Autodesk Inventor part; units mm, degrees
ref_plane "YZ Plane" through (0, 0, 0) normal (1, 0, 0) x (0, 1, 0)
ref_plane "XZ Plane" through (0, 0, 0) normal (0, 1, 0) x (-1, 0, 0)
ref_plane "XY Plane" through (0, 0, 0) normal (0, 0, 1) x (1, 0, 0)
ref_plane "Arbeitsebene1" through (8.2312, -3.2392, 2) normal (0, 0, 1) x (1, 0, 0)
sketch "Skizze1" plane through (8.2312, -3.2392, 2) normal (0, 0, 1) x (1, 0, 0)
  arc A0 (-29.666, 52.3362) -> (-30.2278, 49.15) centre (-26.4114, 50.1197) ccw
  line L0 (-30.4697, 49.0886) -> (-31.8651, 51.0813)
  line L1 (-27.3731, 44.6661) -> (-28.7684, 46.6589)
  line L2 (-25.3803, 46.0614) -> (-27.3731, 44.6661)
  spline S0 degree 3 poles (-25.3803, 46.0614) (-25.4758, 46.0372) (-25.5717, 46.0164) (-25.765, 45.9815) (-25.8623, 45.9675) (-25.9823, 45.9545) (-26.0046, 45.9522) (-26.0633, 45.9468) (-26.0993, 45.944) (-26.1701, 45.9393) (-26.2048, 45.9374) (-26.2421, 45.9359) (-26.244, 45.9358) (-26.3578, 45.9313) (-26.4696, 45.9314) (-26.6928, 45.9405) (-26.8042, 45.9495) (-26.9899, 45.972) (-27.0643, 45.983) (-27.2355, 46.0132) (-27.3315, 46.0336) (-27.5218, 46.0812) (-27.6161, 46.1083) (-27.7358, 46.1473) (-27.7619, 46.1561) (-27.8204, 46.1765) (-27.8532, 46.1884) (-27.9183, 46.2129) (-27.9507, 46.2255) (-27.9876, 46.2405) (-27.9928, 46.2426) (-28.0892, 46.282) (-28.1788, 46.3225) (-28.3547, 46.4094) (-28.4411, 46.456) (-28.6083, 46.5538) (-28.6891, 46.6048) (-28.7684, 46.6589) knots 0 0 0 0 0.084049 0.084049 0.16831 0.16831 0.1875 0.1875 0.21875 0.21875 0.248427 0.248427 0.25 0.25 0.343462 0.343462 0.437098 0.437098 0.5 0.5 0.582124 0.582124 0.664424 0.664424 0.6875 0.6875 0.716281 0.716281 0.74522 0.74522 0.75 0.75 0.834095 0.834095 0.918237 0.918237 1 1 1 1
  line L3 (-20.9578, 49.1581) -> (-22.9506, 47.7627)
  line L4 (-22.3532, 51.1509) -> (-20.9578, 49.1581)
  spline S1 degree 3 poles (-22.3532, 51.1509) (-22.3289, 51.0554) (-22.3081, 50.9594) (-22.2732, 50.7662) (-22.2592, 50.6689) (-22.2462, 50.5488) (-22.244, 50.5265) (-22.2385, 50.4679) (-22.2357, 50.4318) (-22.231, 50.3611) (-22.2292, 50.3263) (-22.2276, 50.289) (-22.2276, 50.2871) (-22.2231, 50.1733) (-22.2231, 50.0616) (-22.2322, 49.8384) (-22.2412, 49.727) (-22.2637, 49.5413) (-22.2747, 49.4668) (-22.3049, 49.2957) (-22.3254, 49.1997) (-22.3729, 49.0094) (-22.4, 48.915) (-22.4391, 48.7954) (-22.4479, 48.7693) (-22.4682, 48.7107) (-22.4801, 48.678) (-22.5046, 48.6128) (-22.5173, 48.5804) (-22.5322, 48.5436) (-22.5343, 48.5384) (-22.5738, 48.442) (-22.6142, 48.3524) (-22.7012, 48.1764) (-22.7477, 48.09) (-22.8455, 47.9229) (-22.8966, 47.842) (-22.9506, 47.7627) knots 0 0 0 0 0.084049 0.084049 0.16831 0.16831 0.1875 0.1875 0.21875 0.21875 0.248427 0.248427 0.25 0.25 0.343462 0.343462 0.437098 0.437098 0.5 0.5 0.582124 0.582124 0.664424 0.664424 0.6875 0.6875 0.716281 0.716281 0.74522 0.74522 0.75 0.75 0.834095 0.834095 0.918237 0.918237 1 1 1 1
  line L5 (-25.4498, 55.5734) -> (-24.0545, 53.5806)
  line L6 (-27.4426, 54.178) -> (-25.4498, 55.5734)
  spline S2 degree 3 poles (-27.4426, 54.178) (-27.3471, 54.2023) (-27.2511, 54.2231) (-27.0579, 54.2579) (-26.9606, 54.272) (-26.8406, 54.285) (-26.8183, 54.2872) (-26.7596, 54.2926) (-26.7236, 54.2955) (-26.6528, 54.3001) (-26.6181, 54.302) (-26.5807, 54.3035) (-26.5789, 54.3036) (-26.4651, 54.3081) (-26.3533, 54.308) (-26.1301, 54.299) (-26.0187, 54.29) (-25.833, 54.2675) (-25.7586, 54.2564) (-25.5874, 54.2262) (-25.4914, 54.2058) (-25.3011, 54.1582) (-25.2067, 54.1311) (-25.0871, 54.0921) (-25.061, 54.0833) (-25.0025, 54.0629) (-24.9697, 54.0511) (-24.9046, 54.0266) (-24.8722, 54.0139) (-24.8353, 53.999) (-24.8301, 53.9969) (-24.7337, 53.9574) (-24.6441, 53.917) (-24.4681, 53.83) (-24.3817, 53.7835) (-24.2146, 53.6857) (-24.1337, 53.6346) (-24.0545, 53.5806) knots 0 0 0 0 0.084049 0.084049 0.16831 0.16831 0.1875 0.1875 0.21875 0.21875 0.248427 0.248427 0.25 0.25 0.343462 0.343462 0.437098 0.437098 0.5 0.5 0.582124 0.582124 0.664424 0.664424 0.6875 0.6875 0.716281 0.716281 0.74522 0.74522 0.75 0.75 0.834095 0.834095 0.918237 0.918237 1 1 1 1
  line L7 (-27.0245, 40.5346) -> (-35.6282, 52.8219)
  line L8 (-35.6282, 52.8219) -> (-25.7984, 59.7048)
  line L9 (-25.7984, 59.7048) -> (-17.1947, 47.4175)
  line L10 (-17.1947, 47.4175) -> (-27.0245, 40.5346)
  line L11 (-27.0245, 40.5346) -> (-25.7984, 59.7048) construction
  line L12 (-35.6282, 52.8219) -> (-17.1947, 47.4175) construction
  line L13 (-27.0245, 40.5346) -> (-12.0245, 40.5346) construction
  circle A1 centre (-26.4114, 50.1197) radius 4.5
  circle A2 centre (-26.4114, 50.1197) radius 3.95
  point P0 (-8.2312, 3.2392)
  point P1 (-24.4756, 54.182)
  point P2 (-21.932, 50.5494)
  point P3 (-22.3491, 48.1839)
  point P4 (-25.9817, 45.6403)
  point P5 (-28.3473, 46.0574)
  point P6 (-26.8411, 54.5992)
  dimension "d0" = 125
  dimension "d1" = 15
  dimension "d2" = 12
  dimension "d3" = 9
  dimension "d16" = 7.9
extrude "Extrusion1" add sketch "Skizze1" along normal mid plane 2 contours L1 A1 L2 | A1 L6 S2 L5 L4 S1 L3 L2 S0 L1 | L1 S0 L2 A1 | A1 L4 L3 | L3 S1 L4 A1 | A1 L5 S2 L6 | L6 L5 A1 | L7 L8 L9 L10 | A2
sketch "Skizze2" plane through (-17.5671, 56.4656, 3) normal (0.819152, 0.5735764, 0) x (0, 0, -1)
  line L0 (2, 0) -> (2, -15)
  line L1 (2, 0) -> (0, 0)
  line L2 (0, -15) -> (0, 0)
  line L3 (0, -15) -> (2, -15)
  line L4 (2, 0) -> (2, -15)
  line L5 (2, -15) -> (8.3, -15)
  line L6 (8.3, -15) -> (8.3, -13.5)
  line L7 (8.3, -13.5) -> (6.3, -12.5)
  line L8 (6.3, -12.5) -> (6.3, -13.5)
  line L9 (6.3, -13.5) -> (2, -13.5)
  line L10 (6, -33.1362) -> (6, 10.1688)
  point P0 (3, -56.33)
  point P1 (2, -13.5)
  dimension "d6" = 1.5
  dimension "d7" = 0
  dimension "d8" = 1
  dimension "d9" = 0.3
  dimension "d10" = 2
extrude "Extrusion2" add sketch "Skizze2" against normal up to surface (12 mm away) contours L9 L10 L5 L0 | L9 L8 L7 L6 L5 L10
chamfer "Fase1" distance 2 angle 45 1 edges at (-14.7388, 41.9656, 1)
ref_plane "Arbeitsebene2" through (-13.2653, 50.322, -5.3) normal (0.5735764, -0.819152, 0) x (0.819152, 0.5735764, 0)
mirror "Spiegeln1" about plane through (-13.2653, 50.322, -5.3) normal (0.5735764, -0.819152, 0) of "Extrusion2", "Fase1"
sketch "Skizze3" plane through (-27.3969, 49.5827, 3) normal (-0.5735764, 0.819152, 0) x (0.819152, 0.5735764, 0)
  line L0 (0, 8.3) -> (0, 0)
  line L1 (12, 8.3) -> (12, 0)
  line L2 (0, 8.3) -> (3.2, 8.3)
  line L3 (3.2, 8.3) -> (3.2, 2)
  line L4 (3.2, 2) -> (0, 2)
  line L5 (0, 2) -> (0, 8.3)
  line L6 (12, 8.3) -> (8.8, 8.3)
  line L7 (8.8, 8.3) -> (8.8, 2)
  line L8 (8.8, 2) -> (12, 2)
  line L9 (12, 2) -> (12, 8.3)
  point P0 (-5.9972, 3)
  point P1 (12, 2)
  point P2 (0, 2)
  dimension "d19" = 3.2
  dimension "d20" = 3.2
extrude "Extrusion3" cut sketch "Skizze3" against normal through all
properties part number "Omniscope_Camera_fix"
Read the model definition and answer for the solid it produces. Units are mm, in the model's axes. A direction names the side the tool comes from. Give positions to 0.01 mm unless a question says otherwise; leave off trailing zeros. Loops run counter-clockwise (first coordinate to the right, second up) from the corner with the lowest first, then second, coordinate; pieces in that order, holes last.
Item 1: The part is cut by section C-C (z = -2.25). Write down the section's boundary in (x, y).
Item 2: For faces 5 (the flat face through (-12.156, 43.159, -2.194)), 6 (the flat face through (-15, 43, 0)), 7 (the flat face through (-24.23, 50.64, -2.19)), determine the directions among +Z, -Z, +X, -X, +Y, -Y from which every point of the face is accessible in a straight line to the end or side of a thin tool.
Item 3: Find the intervals of material crossed by line 1 along Z through (x, y) = (-22.75, 43.25); line 2 along X through (y, z) = (42.5, -4.25); line 3 along Y through (x, z) = (-21.5, -2.25), in increasing order.
Item 4: The mould has two halves that part along Z. Classify faces 1 (the flat face through (-16.744, 39.947, -2.194)), 2 (the flat face through (-21.59, 51.82, -2.13)), 3 (the flat face through (-18, 47, 3)), 4 (the flat face through (-14, 41, -5.3)): released by +Z, released by -Z, zero draft, split by the parting line, or undercut.
Item 5: The part is cut by section B-B (x = -20.5). Write down the section's boundary in (y, z), and give its area (3 significant figures).
Item 6: The part is cut by section A-A (z = -4.5). Write down the section's boundary in (x, y), and give its area (3 significant figures).
Item 7: The part is cut by section D-D (y = 52.25). Write down the section's boundary in (x, z).
Item 8: Each of these flat-tipped pins is pushed along its axis until it touches: pin 1 Ø1.5 at (x, y) = (-22.5, 47) entering from -Z; pin 2 Ø1.5 at (y, z) = (54, 1) entering from +X; pin 3 Ø3 at (x, z) = (-18.5, 2) entering from -Y; pin 4 Ø1.5 at (x, z) = (-23, -0.5) entering from +Y. Where does it stop, or does it pass through?
Taken from the geometry:
1. outline: (-24.78, 51.42) - (-23.92, 50.19) - (-19.33, 53.4) - (-20.19, 54.63) - close; (-17.03, 40.36) - (-16.17, 39.13) - (-11.58, 42.34) - (-12.45, 43.57) - close
2. face 5: -Z, +X, +Y
2. face 6: -X, +Y
2. face 7: -Z, -X, -Y
3. line 1: z = 1 to 3
3. line 2: x = -14.89 to -11.69
3. line 3: y = 51.88 to 53.71
4. face 1: zero draft
4. face 2: undercut
4. face 3: released by +Z
4. face 4: released by -Z
5. outline: (39.73, 1) - (50.14, 1) - (52.58, -1) - (52.58, -3.3) - (51.36, -3.3) - (52.58, -5.3) - (54.41, -5.3) - (54.41, 3) - (39.73, 3) - close
5. area: 44.6 mm2
6. outline: (-24.78, 51.42) - (-23.69, 49.86) - (-19.1, 53.07) - (-20.19, 54.63) - close; (-17.26, 40.69) - (-16.17, 39.13) - (-11.58, 42.34) - (-12.67, 43.9) - close
6. area: 21.3 mm2
7. outline: (-23.59, -5.3) - (-20.97, -5.3) - (-19.23, -3.3) - (-20.97, -3.3) - (-20.97, -1) - (-18.52, 0.41) - (-18.52, 1) - (-14.62, 1) - (-14.62, 3) - (-23.59, 3) - close
8. pin 1: stops at z = 1
8. pin 2: stops at x = -15.32
8. pin 3: stops at y = 37.3
8. pin 4: stops at y = 53.19
